Input: dimensioned drawing with shaded views. Units: mm. Origin: part minimum x, y, z. A direction names the side the tool comes from. Coordinates: 2 decimals unless noted, no trailing zeros. Order: outer loops, then holes, each group sorted by start corner. A loop starts at its lowest first (then second) coordinate and runs counter-clockwise, first axis right, second up. Notation, with made-up numbers: (69.25, 6.25) -> (80.25, 6.25) arc R26 cw to (80.25, 42.25) -> close; hole circle Ø9 at (-16.75, -32.75). An arc over 180 degrees is marked (long way). Answer as CSV lines item,"result".
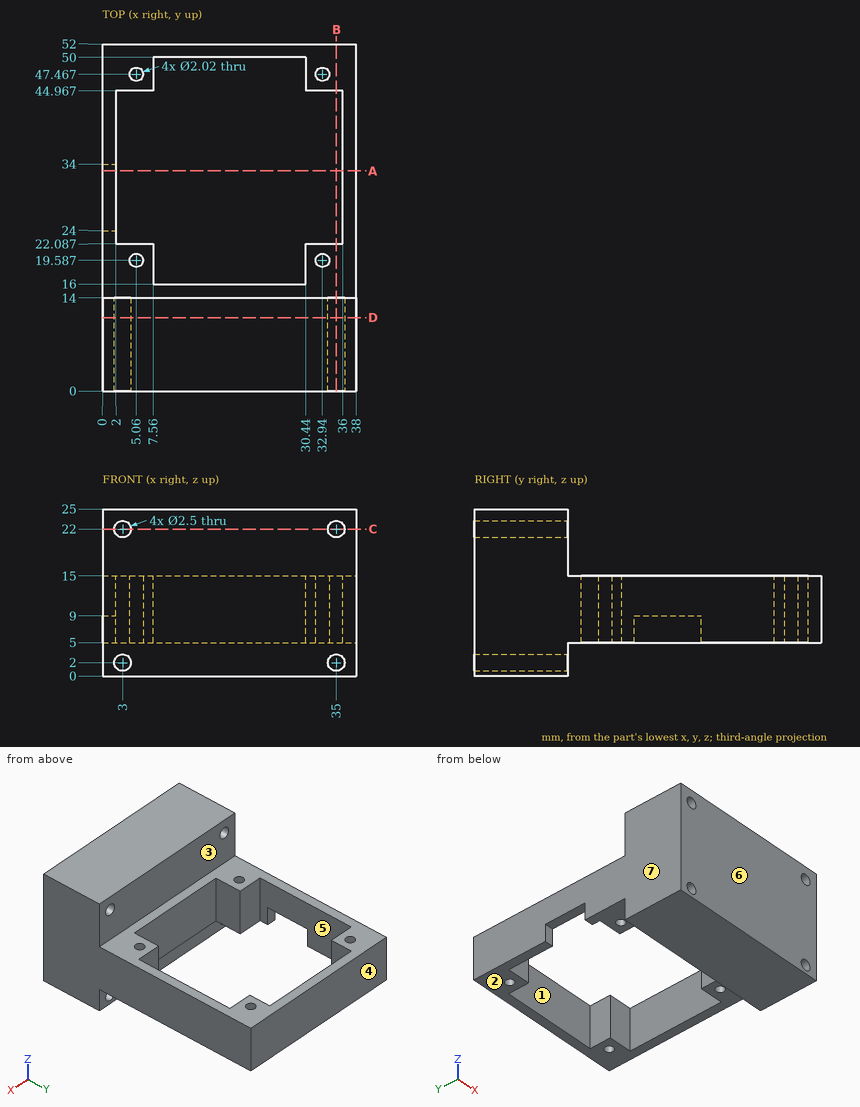
1. Cut plane A-A (y = 33). Return the cut outline in (x, z).
Findings:
outline,"(0, 9) -> (2, 9) -> (2, 15) -> (0, 15) -> close; (36, 5) -> (38, 5) -> (38, 15) -> (36, 15) -> close"
2. Cut plane D-D (y = 11). Return the cut outline in (x, z), plus the area to 3 significant figures.
Findings:
outline,"(0, 0) -> (38, 0) -> (38, 25) -> (0, 25) -> close; hole circle Ø2.5 at (3, 2); hole circle Ø2.5 at (3, 22); hole circle Ø2.5 at (35, 2); hole circle Ø2.5 at (35, 22)"
area,"930 mm2"
3. Cut plane B-B (x = 35). Return the cut outline in (y, z).
Findings:
outline,"(0, 0) -> (14, 0) -> (14, 0.75) -> (0, 0.75) -> close; (0, 3.25) -> (14, 3.25) -> (14, 5) -> (22.09, 5) -> (22.09, 15) -> (14, 15) -> (14, 20.75) -> (0, 20.75) -> close; (0, 23.25) -> (14, 23.25) -> (14, 25) -> (0, 25) -> close; (44.97, 5) -> (52, 5) -> (52, 15) -> (44.97, 15) -> close"
4. Reachability of the marked faces 1, 2, 3 and 4 from +Z, -Z, +X, -X, +Y, -Y: full face, straight path, thin tool, end or side. Return the list, or none.
Findings:
face 1,"+Z, -Z"
face 2,"-Z, +X, -X, +Y"
face 3,"+Z, +X, -X, +Y"
face 4,"+Z, -Z, +X, -X, +Y"
5. Mould query, pull axis X, two halves, no side actions, for the marked faces 5, 6 and 7. Classes: released by +X, released by -X, zero draft, split by the parting line, or undercut.
Findings:
face 5,"undercut"
face 6,"zero draft"
face 7,"released by -X"
6. Ray query, line 1 along Y through (x, z) = (32.94, 10.5); line 2 along X through (y, z) = (19.5, 7.5); line 3 along X through (y, z) = (7, 2). Return the intervals inside material, ascending.
Findings:
line 1,"y = 0 to 18.58, 20.6 to 22.09, 44.97 to 46.46, 48.48 to 52"
line 2,"x = 0 to 4.05, 6.07 to 7.56, 30.44 to 31.93, 33.95 to 38"
line 3,"x = 0 to 1.75, 4.25 to 33.75, 36.25 to 38"
7. Cut plane C-C (z = 22). Return the cut outline in (x, y).
Findings:
outline,"(0, 0) -> (1.75, 0) -> (1.75, 14) -> (0, 14) -> close; (4.25, 0) -> (33.75, 0) -> (33.75, 14) -> (4.25, 14) -> close; (36.25, 0) -> (38, 0) -> (38, 14) -> (36.25, 14) -> close"
8. Contact query for flat-ended pins moving along their axis: pin 1 (1.6 mm diameter, centred on x = 1.5, y = 29.5, fed in from -Z); pin 2 (4 mm diameter, centred on x = 3, z = 22, fed in from +Y); pin 3 (2 mm diameter, centred on x = 35, z = 22, fed in from +Y); pin 4 (2.5 mm diameter, centred on x = 5.06, y = 19.59, fed in from +Z). Output: stop coordinate, or through.
Findings:
pin 1,"stops at z = 9"
pin 2,"stops at y = 14"
pin 3,"passes through"
pin 4,"stops at z = 15"
